```python
from build123d import *

# Parameters (mm, degrees)
SKETCH1_W           = 56
SKETCH1_H           = 50
BOSS_EXTRUDE1_DEPTH = 3
SKETCH2_R           = 1.5
CUT_EXTRUDE1_DEPTH  = 76.133215025
SKETCH3_W           = 12
SKETCH3_H           = 3
BOSS_EXTRUDE2_DEPTH = 26
SKETCH5_R           = 1.5
CUT_EXTRUDE2_DEPTH  = 10
BOSS_EXTRUDE3_DEPTH = 3
SKETCH7_W           = 2
SKETCH7_H           = 7.5
BOSS_EXTRUDE4_DEPTH = 10
SKETCH8_R           = 1.5
CUT_EXTRUDE3_DEPTH  = 69.900290275
FILLET1_R           = 2.5
FILLET2_R           = 2.5
FILLET3_R           = 2.5
FILLET4_R           = 2.5


with BuildPart() as part:
    # Sketch1 → Boss-Extrude1 (new body)
    with BuildSketch(Plane.XY):
        with Locations((28, 25)):
            Rectangle(SKETCH1_W, SKETCH1_H)
    extrude(amount=BOSS_EXTRUDE1_DEPTH)

    # Sketch2 → Cut-Extrude1 (cut, through all)
    with BuildSketch(Plane.XY.offset(3)):
        with Locations((18, 10)):
            Circle(SKETCH2_R)
        with Locations((18, 45)):
            Circle(SKETCH2_R)
        with Locations((53, 45)):
            Circle(SKETCH2_R)
        with Locations((53, 10)):
            Circle(SKETCH2_R)
        with Locations((6, 6)):
            Circle(SKETCH2_R)
        with Locations((6, 41)):
            Circle(SKETCH2_R)
    extrude(amount=-CUT_EXTRUDE1_DEPTH, mode=Mode.SUBTRACT)

    # Sketch3 → Boss-Extrude2 (add)
    with BuildSketch(Plane.XY.offset(3)):
        with Locations((6, 21.5)):
            Rectangle(SKETCH3_W, SKETCH3_H)
    extrude(amount=BOSS_EXTRUDE2_DEPTH)

    # Sketch5 → Cut-Extrude2 (cut)
    with BuildSketch(Plane(origin=(0, 23, 0), x_dir=(1, 0, 0), z_dir=(0, 1, 0))):
        with Locations(Location((6, -7, 0), (0, 0, 270))):
            Circle(SKETCH5_R)
        with Locations(Location((6, -25, 0), (0, 0, 270))):
            Circle(SKETCH5_R)
    extrude(amount=-CUT_EXTRUDE2_DEPTH, mode=Mode.SUBTRACT)

    # Sketch6 → Boss-Extrude3 (add)
    with BuildSketch(Plane(origin=(12, 0, 0), x_dir=(0, 0, -1), z_dir=(1, 0, 0))):
        Polygon((-3, 20), (-29, 20), (-29, 23), (-13, 42.5), (-3, 42.5), align=None)
    extrude(amount=BOSS_EXTRUDE3_DEPTH)

    # Sketch7 → Boss-Extrude4 (add)
    with BuildSketch(Plane.XY.offset(3)):
        with Locations((19.5, 3.75)):
            Rectangle(SKETCH7_W, SKETCH7_H)
        with Locations((51.5, 3.75)):
            Rectangle(SKETCH7_W, SKETCH7_H)
    extrude(amount=BOSS_EXTRUDE4_DEPTH)

    # Sketch8 → Cut-Extrude3 (cut, through all)
    with BuildSketch(Plane.ZY.offset(-18.5)):
        with Locations((8, 3)):
            Circle(SKETCH8_R)
    extrude(amount=-CUT_EXTRUDE3_DEPTH, mode=Mode.SUBTRACT)

    # Fillet1
    fillet1_edges = [part.edges().sort_by_distance(p)[0] for p in [
        (0, 50, 1.5),
        (56, 50, 1.5),
        (56, 0, 1.5),
        (0, 0, 1.5),
    ]]
    fillet(fillet1_edges, radius=FILLET1_R)

    # Fillet2
    fillet2_edges = [part.edges().sort_by_distance(p)[0] for p in [
        (6, 23, 3),
        (12, 23, 16),
        (12, 32.75, 3),
        (18.5, 3.75, 3),
        (52.5, 3.75, 3),
    ]]
    fillet(fillet2_edges, radius=FILLET2_R - 0.0001)  # a hair under: the kernel refuses the full size

    # Fillet3
    fillet3_edges = [part.edges().sort_by_distance(p)[0] for p in [
        (0, 21.5, 29),
        (15, 21.5, 29),
    ]]
    fillet(fillet3_edges, radius=FILLET3_R)

    # Fillet4
    fillet4_edges = [part.edges().sort_by_distance(p)[0] for p in [
        (19.5, 0, 13),
        (51.5, 0, 13),
    ]]
    fillet(fillet4_edges, radius=FILLET4_R)


solid = part.part
```
Design review of the part built by this model. Coordinates are the model's own, in mm. A direction names the side the tool comes from. Give positions to 0.01 mm unless a question says otherwise; leave off trailing zeros. Loops run counter-clockwise (first coordinate to the right, second up) from the corner with the lowest first, then second, coordinate; pieces in that order, holes last. Notation, with made-up numbers: (-40, 51) -> (-8, 51) arc R29 cw to (-8, 81) -> close; hole circle Ø10 at (14, 88.25). An arc over 180 degrees is marked (long way). One line per item, written item: value.
Q1. Draft analysis for pull direction Z (two halves, no side actions). For faces 6 (the cylindrical face through (19.5, 2.1, 6.8)), 7 (the flat face through (28, 25, 0)), 8 (the cylindrical face through (14.564, 22.394, 27.911)), state which applies: pulls with the +Z half, pulls with the -Z half, needs draft (parallel to the pull), parting line crosses it, or undercut.
Numbers:
face 6: undercut
face 7: pulls with the -Z half
face 8: pulls with the +Z half
Q2. We need section D-D on x = 39.5. Give the boundary of the cut face in (y, z).
Numbers:
outline: (0, 0) -> (50, 0) -> (50, 3) -> (0, 3) -> close
Q3. We need section B-B on z = 7.5. Give the boundary of the cut face in (x, y), and give its area (3 significant figures).
Numbers:
outline: (0, 20) -> (4.59, 20) -> (4.59, 23) -> (0, 23) -> close; (7.41, 20) -> (15, 20) -> (15, 42.5) -> (12, 42.5) -> (12, 25.5) arc R2.5 cw to (9.5, 23) -> (7.41, 23) -> close; (18.5, 0) -> (20.5, 0) -> (20.5, 1.59) -> (18.5, 1.59) -> close; (18.5, 4.41) -> (20.5, 4.41) -> (20.5, 7.5) -> (18.5, 7.5) -> close; (50.5, 0) -> (52.5, 0) -> (52.5, 1.59) -> (50.5, 1.59) -> close; (50.5, 4.41) -> (52.5, 4.41) -> (52.5, 7.5) -> (50.5, 7.5) -> close
area: 115 mm^2
Q4. For pin 1 Ø2 at (x, y) = (20, 5.5) entering from +Z; pin 2 Ø1.3 at (x, z) = (18.5, 8) entering from +Y; pin 3 Ø1.8 at (x, y) = (18, 10) entering from -Z; pin 4 Ø3.5 at (y, z) = (3, 8) entering from +X, all flat-tipped, find the tip position at first contact; note any pin that passes through.
Numbers:
pin 1: stops at z = 13
pin 2: stops at y = 7.5
pin 3: passes through
pin 4: stops at x = 52.5
Q5. We need section A-A on y = 45. Give the boundary of the cut face in (x, z).
Numbers:
outline: (0, 0) -> (16.5, 0) -> (16.5, 3) -> (0, 3) -> close; (19.5, 0) -> (51.5, 0) -> (51.5, 3) -> (19.5, 3) -> close; (54.5, 0) -> (56, 0) -> (56, 3) -> (54.5, 3) -> close
Q6. Machinability: for faces 1 (the flat face through (18.5, 5, 9)), 2 (the flat face through (19, 7.5, 8)), 3 (the flat face through (52.5, 5, 9)), 4 (the flat face through (51, 5, 13)), 5 (the flat face through (12, 32, 14)), which of the approach directions +Z, -Z, +X, -X, +Y, -Y give a long, thin tool a straight path to every point of the face, cutting with its end or side? Answer none if there is none.
Numbers:
face 1: +Z, -X, +Y, -Y
face 2: +Z, +X, -X, +Y
face 3: +Z, +X, +Y, -Y
face 4: +Z, +X, -X, +Y, -Y
face 5: +Z, -X, +Y
Q7. For L1, parallel to Y at x = 6, z = 1.85; L2, parallel to X at y = 21.3, z = 7; L3, parallel to Y at x = 53, z = 1.05, list the stretches that pass through material, from the lowest coordinate up.
Numbers:
L1: y = 0 to 4.5, 7.5 to 39.5, 42.5 to 50
L2: x = 0 to 4.5, 7.5 to 15
L3: y = 0 to 8.5, 11.5 to 43.5, 46.5 to 50
Q8. We need section C-C on z = 25. Give the boundary of the cut face in (x, y) (3 decimals), and give its area (3 significant figures).
Numbers:
outline: (0, 20) -> (4.5, 20) -> (4.5, 23) -> (0, 23) -> close; (7.5, 20) -> (15, 20) -> (15, 27.875) -> (12, 27.875) -> (12, 25.5) arc R2.5 cw to (9.5, 23) -> (7.5, 23) -> close
area: 52.0 mm^2
